Design review of the part built by this model. Coordinates are the model's own, in mm. Face numbers are marked on the shaded views. A direction names the side the tool comes from. Coordinates: 2 decimals unless noted, no trailing zeros. Write each loop counter-clockwise with the first axis right and the second up, starting at its lowest first coordinate (ties: lowest second). Pieces come first, ordered by that corner, then holes. Notation, with made-up numbers: (52.25, 1) - (57.25, 1) arc R18 cw to (57.25, 6) - close; hole circle Ø4 at (-26, 73). An arc over 180 degrees is marked (long way). Answer as a JSON object with one key per item and string values.
Autodesk Inventor part; units mm, degrees
ref_plane "YZ Plane" through (0, 0, 0) normal (1, 0, 0) x (0, 1, 0)
ref_plane "XZ Plane" through (0, 0, 0) normal (0, 1, 0) x (-1, 0, 0)
ref_plane "XY Plane" through (0, 0, 0) normal (0, 0, 1) x (1, 0, 0)
sketch "Sketch1" plane through (0, 0, 0) normal (0, 1, 0) x (-1, 0, 0)
  circle A0 centre (0, 0) radius 2.5
  circle A1 centre (0, 0) radius 5.5
  line L0 (5.5, 5.5) -> (-5.5, 5.5)
  line L1 (-5.5, 5.5) -> (-5.5, 6.5)
  line L2 (-5.5, 6.5) -> (5.5, 6.5)
  line L3 (5.5, 6.5) -> (5.5, 5.5)
  line L4 (0, -7.9) -> (0, 8.9) construction
  line L5 (0, 0) -> (-5.5, 3.175426)
  line L6 (0, 0) -> (-5.5, 0)
  line L7 (5.5, 0) -> (5.5, 5.5)
  line L8 (-5.5, 0) -> (-5.5, 5.5)
  point P0 (-2.5, 0)
  point P1 (0, 5.5)
  point P2 (-2.165064, 1.25)
  dimension "d0" = 5
  dimension "d1" = 3
  dimension "d4" = 30
  dimension "d5" = 1
sketch "Sketch1 outline for Extrusion1" plane through (0, 0, 0) normal (0, 1, 0) x (-1, 0, 0)
  line L0 (5.5, 0) -> (5.5, 6.5)
  line L1 (5.5, 6.5) -> (-5.5, 6.5)
  line L2 (-5.5, 6.5) -> (-5.5, 3.175426)
  line L3 (-5.5, 3.175426) -> (-2.165064, 1.25)
  arc A0 (-2.165064, 1.25) -> (-2.5, 0) centre (0, 0) cw
  line L4 (-2.5, 0) -> (-5.5, 0)
  arc A1 (-5.5, 0) -> (5.5, 0) centre (0, 0) ccw
extrude "Extrusion1" add sketch "Sketch1 outline for Extrusion1" along normal blind 15
fillet "Fillet1" radius 2 4 edges at (5.5, 7.5, 3.1754) (2.1651, 7.5, 1.25) (2.5, 7.5, 0) (5.5, 7.5, 0)
properties part number "Cable Clip"
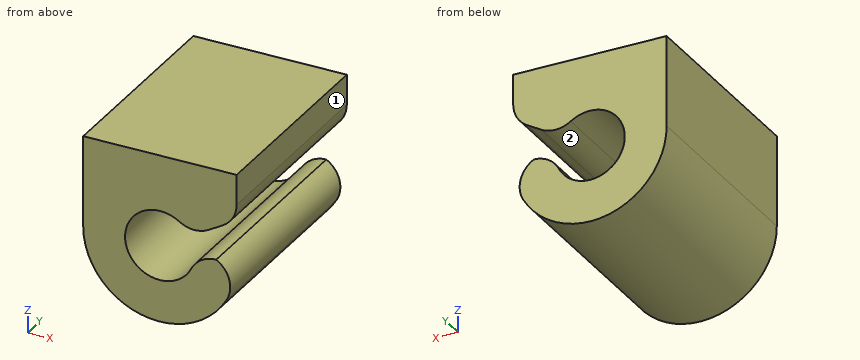
(1) Take a section at D-D, the plane x = -3.5. Write out the cut boundary in (y, z).
Solved:
{"outline": "(0, -4.24) - (15, -4.24) - (15, 6.5) - (0, 6.5) - close"}
(2) Take a section at A-A, the plane x = 0. Write out the cut boundary in (y, z), and give its area (3 significant figures).
Solved:
{"outline": "(0, -5.5) - (15, -5.5) - (15, -2.5) - (0, -2.5) - close; (0, 2.5) - (15, 2.5) - (15, 6.5) - (0, 6.5) - close", "area": "105 mm^2"}
(3) Take a section at B-B, the plane z = -1.5. Write out the cut boundary in (x, y).
Solved:
{"outline": "(-5.29, 0) - (-2, 0) - (-2, 15) - (-5.29, 15) - close; (2, 0) - (5.02, 0) - (5.02, 15) - (2, 15) - close"}
(4) To check wall thickness, follow line 1 (Z direction, x = 0, y = 9.5); line 2 (Z direction, x = 2, y = 9.5); line 3 (X direction, y = 11.75, z = 2.25). State the ranges of each line that lie inside material, in increasing order. Write a range as from..to.
Solved:
{"line 1": "z = -5.5..-2.5, 2.5..6.5", "line 2": "z = -5.12..-1.5, 1.81..6.5", "line 3": "x = -5.5..-1.09, 1.09..3.9"}
(5) For pin 1 (3 mm diameter, centred on y = 11.5, z = 0, fed in from +X), flat-tipped, find the tip position at first contact; note if it passes through.
Solved:
{"pin 1": "stops at x = 5.02"}
(6) Tool access review of the marked faces 1 and 2: name each direction out of +Z, -Z, +X, -X, +Y, -Y from which nothing blocks a thin tool from reaching the whole face with its end or side.
Solved:
{"face 1": "+Z, -Z, +X, +Y, -Y", "face 2": "+Y, -Y"}
(7) Take a section at C-C, the plane y = 3.25. Write out the cut boundary in (x, z).
Solved:
{"outline": "(-5.5, 0) arc R5.5 ccw to (4.78, -2.73) arc R2 ccw to (4.03, 0) arc R2 ccw to (2.24, -1.11) arc R2.5 cw (long way) to (1.38, 2.08) arc R2 ccw to (3.49, 2.02) - (4.5, 2.6) arc R2 ccw to (5.5, 4.33) - (5.5, 6.5) - (-5.5, 6.5) - close"}
